For this review, use the dimensioned drawing (mm, ordinates from the lowest corner) and the shaded views. Coordinates: 2 decimals unless noted, no trailing zeros. Write each loop counter-clockwise with the first axis right and the second up, starting at its lowest first coordinate (ties: lowest second). Pieces come first, ordered by that corner, then holes. Notation, with made-up numbers: (1, 24.5) - (30, 24.5) arc R10 ccw to (30, 43.5) - close; hole circle Ø7 at (-12.75, 3.5). An arc over 180 degrees is marked (long way). Answer as a JSON object with one key per item and string values.
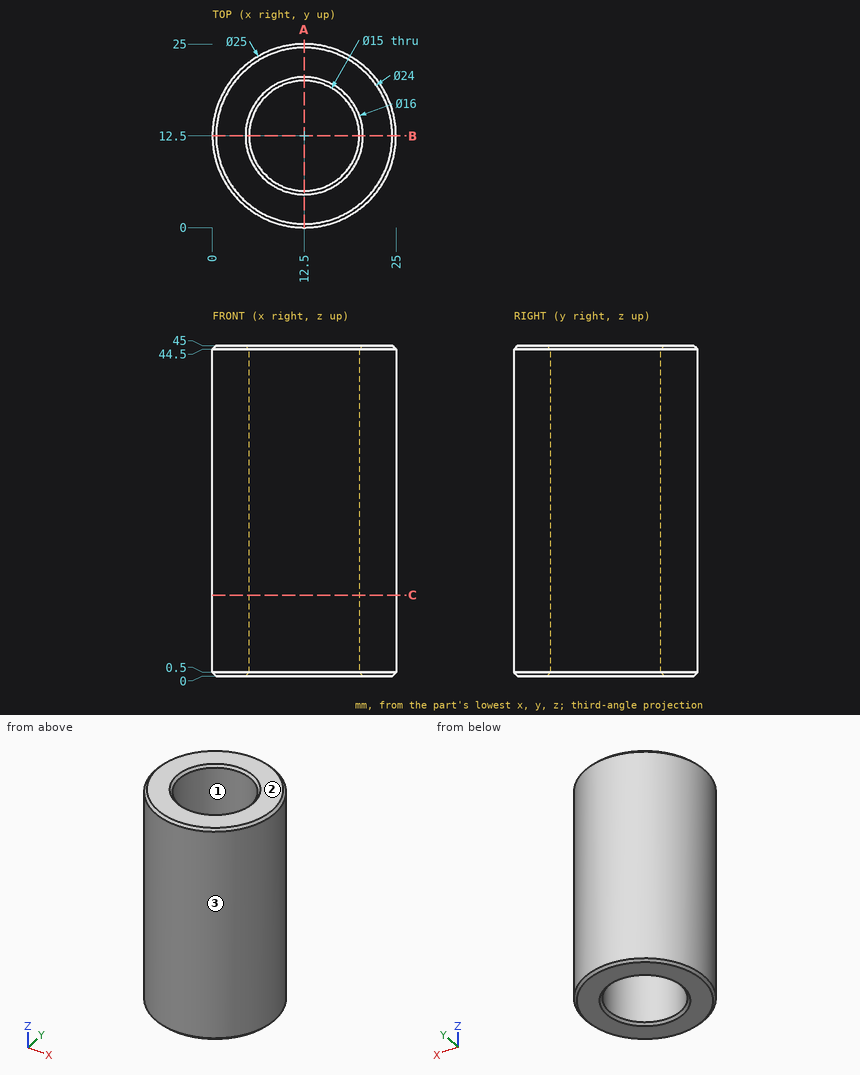
(1) Take a section at A-A, the plane x = 12.5. Write out the cut boundary in (y, z).
Solved:
{"outline": "(0, 0.5) - (0.5, 0) - (4.5, 0) - (5, 0.5) - (5, 44.5) - (4.5, 45) - (0.5, 45) - (0, 44.5) - close; (20, 0.5) - (20.5, 0) - (24.5, 0) - (25, 0.5) - (25, 44.5) - (24.5, 45) - (20.5, 45) - (20, 44.5) - close"}
(2) For pin 1 (1 mm diameter, centred on y = 10.5, z = 27, fed in from -X); pin 2 (8 mm diameter, centred on x = 3.5, z = 11, fed in from -Y); pin 3 (1.5 mm diameter, centred on y = 8, z = 11, fed in from +X), all flat-tipped, find the tip position at first contact; note any pin that passes through.
Solved:
{"pin 1": "stops at x = 0.09", "pin 2": "stops at y = 1.04", "pin 3": "stops at x = 24.42"}
(3) To check wall thickness, follow line 1 (Y direction, x = 12.5, z = 34.5); line 2 (Y direction, x = 18, z = 24.5); line 3 (X direction, y = 14, z = 26.5). State the ranges of each line that lie inside material, in increasing order. Write a range as from..to.
Solved:
{"line 1": "y = 0..5, 20..25", "line 2": "y = 1.28..7.4, 17.6..23.72", "line 3": "x = 0.09..5.15, 19.85..24.91"}
(4) The part is to be moulded in two halves that separate along Y. For the marked faces 1, 2 and 3, say which applies: pulls with the +Y half, pulls with the -Y half, needs draft (parallel to the pull), parting line crosses it, or undercut.
Solved:
{"face 1": "undercut", "face 2": "needs draft", "face 3": "parting line crosses it"}
(5) Take a section at C-C, the plane z = 11. Write out the cut boundary in (x, y), and give its area (3 significant figures).
Solved:
{"outline": "circle Ø25 at (12.5, 12.5); hole circle Ø15 at (12.5, 12.5)", "area": "314 mm^2"}
